Design review of the part built by this model. Coordinates are the model's own, in mm. Face numbers are marked on the shaded views. A direction names the side the tool comes from. Coordinates: 2 decimals unless noted, no trailing zeros. Order: outer loops, then holes, each group sorted by start corner. A loop starts at its lowest first (then second) coordinate and runs counter-clockwise, first axis right, second up. Notation, with made-up numbers: (30, 37.25) -> (88, 37.25) arc R32 ccw to (88, 66.25) -> close; hole circle Ø6 at (1.25, 28). An arc over 180 degrees is marked (long way). Write item = value, one per line.
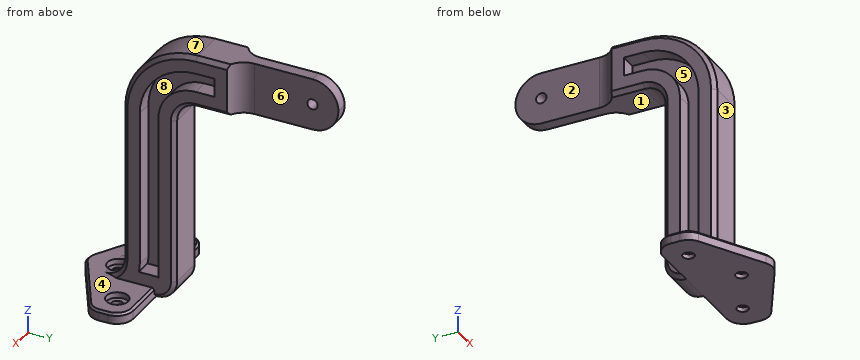
```python
from build123d import *

# Parameters (mm, degrees)
BOSS_EXTRUDE1_DEPTH             = 5
FILLET1_R                       = 8
CBORE_FOR_M5_SBHCS1_D           = 5.5
CBORE_FOR_M5_SBHCS1_DEPTH       = 10
CBORE_FOR_M5_SBHCS1_CBORE_D     = 10.5
CBORE_FOR_M5_SBHCS1_CBORE_DEPTH = 2.75
CBORE_FOR_M5_SBHCS1_TIP         = 1.652366702
SKETCH7_W                       = 20
SKETCH7_H                       = 100
BOSS_EXTRUDE2_DEPTH             = 120
SKETCH8_W                       = 190
SKETCH8_H                       = 150
CUT_EXTRUDE1_DEPTH              = 72
FILLET2_R                       = 12.5
SKETCH9_W                       = 14.25
SKETCH9_H                       = 100
CUT_EXTRUDE2_DEPTH              = 72
SKETCH10_R                      = 2.5
CUT_EXTRUDE3_DEPTH              = 72
FILLET3_R                       = 10
FILLET4_R                       = 10
FILLET5_R                       = 35
FILLET6_R                       = 10
SKETCH12_W                      = 20
SKETCH12_H                      = 10
BOSS_EXTRUDE3_DEPTH             = 5
FILLET7_R                       = 10
CHAMFER1_SIZE                   = 2
CHAMFER2_SIZE                   = 1
CUT_EXTRUDE4_DEPTH              = 8


# Some blends are built 0.0001 mm under size
with BuildPart() as part:
    # Sketch2 → Boss-Extrude1 (new body)
    with BuildSketch(Plane.XY):
        Polygon((-37.5, 28.000635095), (0, 6.35), (37.5, 28.000635095), (37.5, 45), (-37.5, 45), align=None)
    extrude(amount=BOSS_EXTRUDE1_DEPTH)

    # Fillet1
    fillet1_edges = [part.edges().sort_by_distance(p)[0] for p in [
        (37.5, 28.000635095, 2.5),
        (0, 6.35, 2.5),
        (-37.5, 28.000635095, 2.5),
        (-37.5, 45, 2.5),
        (37.5, 45, 2.5),
    ]]
    fillet(fillet1_edges, radius=FILLET1_R)

    # CBORE for M5 SBHCS1
    with Locations(Plane.XY.offset(5)):
        with Locations((-25, 35), (0, 22.5), (25, 35)):
            CounterBoreHole(CBORE_FOR_M5_SBHCS1_D / 2, CBORE_FOR_M5_SBHCS1_CBORE_D / 2, CBORE_FOR_M5_SBHCS1_CBORE_DEPTH, depth=CBORE_FOR_M5_SBHCS1_DEPTH)
            with Locations((0, 0, -(CBORE_FOR_M5_SBHCS1_DEPTH + CBORE_FOR_M5_SBHCS1_TIP / 2))):  # 118° drill point
                Cone(0, CBORE_FOR_M5_SBHCS1_D / 2, CBORE_FOR_M5_SBHCS1_TIP, mode=Mode.SUBTRACT)

    # Sketch7 → Boss-Extrude2 (add)
    with BuildSketch(Plane.XY.offset(5)):
        with Locations((0, 80)):
            Rectangle(SKETCH7_W, SKETCH7_H)
    extrude(amount=BOSS_EXTRUDE2_DEPTH)

    # Sketch8 → Cut-Extrude1 (cut)
    with BuildSketch(Plane(origin=(10, 0, 0), x_dir=(0, 0, -1), z_dir=(1, 0, 0))):
        with Locations((-5, 130)):
            Rectangle(SKETCH8_W, SKETCH8_H)
    extrude(amount=-CUT_EXTRUDE1_DEPTH, mode=Mode.SUBTRACT)

    # Fillet2
    fillet2_edges = [part.edges().sort_by_distance(p)[0] for p in [
        (0, 130, 100),
        (0, 130, 125),
    ]]
    fillet(fillet2_edges, radius=FILLET2_R - 0.0001)  # a hair under: the kernel refuses the full size

    # Sketch9 → Cut-Extrude2 (cut)
    with BuildSketch(Plane.XY.offset(125)):
        with Locations((10, 130)):
            Rectangle(SKETCH9_W, SKETCH9_H)
        with Locations((-10, 130)):
            Rectangle(SKETCH9_W, SKETCH9_H)
    extrude(amount=-CUT_EXTRUDE2_DEPTH, mode=Mode.SUBTRACT)

    # Sketch10 → Cut-Extrude3 (cut)
    with BuildSketch(Plane(origin=(2.875, 0, 0), x_dir=(0, 0, -1), z_dir=(1, 0, 0))):
        with Locations((-112.5, 117.5)):
            Circle(SKETCH10_R)
    extrude(amount=-CUT_EXTRUDE3_DEPTH, mode=Mode.SUBTRACT)

    # Fillet3
    # the kernel refuses this fillet: 10 mm, written as the material it adds along each edge
    with BuildSketch(Plane(origin=(-2.875, 80, 125), x_dir=(-1, 0, 0), z_dir=(0, 0, -1))) as fillet3_piece_1:
        with BuildLine():
            CenterArc((10, 9.577806377), FILLET3_R, 180, 73.291656284)
            Line((0, 9.577806377), (-0.2, 9.577806377))
            Line((-0.2, 9.577806377), (-0.2, 0))
            Line((-0.2, 0), (0, -0.2))
            ThreePointArc((0, -0.2), (3.5625, -0.2), (7.0675, -0.191556128))
            Line((7.0675, -0.191556128), (7.125, 0))
        make_face()
    extrude(amount=25)
    with BuildSketch(Plane(origin=(2.875, 80, 125), x_dir=(0, 1, 0), z_dir=(0, 0, -1))) as fillet3_piece_2:
        with BuildLine():
            CenterArc((9.577806377, 10), FILLET3_R, 196.708343716, 73.291656284)
            Line((0, 7.125), (-0.191556128, 7.0675))
            ThreePointArc((-0.191556128, 7.0675), (-0.2, 3.5625), (-0.2, 0))
            Line((-0.2, 0), (0, -0.2))
            Line((0, -0.2), (9.577806377, -0.2))
            Line((9.577806377, -0.2), (9.577806377, 0))
        make_face()
    extrude(amount=25)

    # Fillet4
    fillet4_edges = [part.edges().sort_by_distance(p)[0] for p in [
        (0, 55, 100),
    ]]
    fillet(fillet4_edges, radius=FILLET4_R)

    # Fillet5
    fillet5_edges = [part.edges().sort_by_distance(p)[0] for p in [
        (0, 30, 125),
    ]]
    fillet(fillet5_edges, radius=FILLET5_R)

    # Fillet6
    # the kernel refuses this fillet: 10 mm, written as the material it adds along each edge
    with BuildSketch(Plane(origin=(10, 30, 5), x_dir=(0, 0, 1), z_dir=(-1, 0, 0))) as fillet6_piece_1_section:
        with BuildLine():
            CenterArc((FILLET6_R, -FILLET6_R), FILLET6_R, 90, 90)
            Line((0, -FILLET6_R), (0, 0))
            Line((0, 0), (FILLET6_R, 0))
        make_face()
    fillet6_piece_1 = extrude(amount=20, mode=Mode.PRIVATE)
    fillet6_piece_1 = fillet6_piece_1 - Plane(origin=(0, 22.5, 7.53044348), x_dir=(1, 0, 0), z_dir=(0, 0, 1)) * Cylinder(5.25, 80, mode=Mode.PRIVATE)
    add(fillet6_piece_1)

    # Sketch12 → Boss-Extrude3 (add)
    with BuildSketch(Plane(origin=(0, 0, 5), x_dir=(-1, 0, 0), z_dir=(0, 0, -1))):
        with Locations((0, 50)):
            Rectangle(SKETCH12_W, SKETCH12_H)
    extrude(amount=BOSS_EXTRUDE3_DEPTH)

    # Fillet7
    # the kernel refuses this fillet: 10 mm, written as the material it takes off along each edge
    with BuildSketch(Plane(origin=(-35, 55, 0), x_dir=(0, 0, 1), z_dir=(1, 0, 0))) as fillet7_piece_1:
        with BuildLine():
            CenterArc((FILLET7_R, FILLET7_R), FILLET7_R, 180, 90)
            Line((0, FILLET7_R), (0, 0))
            Line((0, 0), (FILLET7_R, 0))
        make_face()
    extrude(amount=70, mode=Mode.SUBTRACT)

    # Chamfer1
    # the kernel refuses this chamfer: 2 mm, written as the material it takes off along each edge
    with BuildSketch(Plane(origin=(-10, 65, 100), x_dir=(-0.02749587661058987, 0, 0.9996219169112968), z_dir=(0, 1, 0)), Plane(origin=(10, 85.143365976, 100), x_dir=(0.027495876610586414, 0, 0.9996219169112968), z_dir=(0, -1, 0))) as chamfer1_piece_1:
        Polygon((CHAMFER1_SIZE * 0.999621916911, CHAMFER1_SIZE * 0.0274958766106), (-CHAMFER1_SIZE * 0.0274958766106, CHAMFER1_SIZE * 0.999621916911), (0, 0), align=None)
    extrude(amount=20.143365976, mode=Mode.SUBTRACT)
    with BuildSketch(Plane(origin=(-10, 65, 125), x_dir=(-0.02749587661058987, 0, -0.9996219169112968), z_dir=(0, 1, 0)), Plane(origin=(10, 85.143365976, 125), x_dir=(0.027495876610586414, 0, -0.9996219169112968), z_dir=(0, -1, 0))) as chamfer1_piece_2:
        Polygon((CHAMFER1_SIZE * 0.999621916911, -CHAMFER1_SIZE * 0.0274958766106), (-CHAMFER1_SIZE * 0.0274958766106, -CHAMFER1_SIZE * 0.999621916911), (0, 0), align=None)
    extrude(amount=20.143365976, mode=Mode.SUBTRACT)
    with BuildSketch(Plane(origin=(-10, 55, 10), x_dir=(-0.027495876610589956, -0.9996219169112965, 0), z_dir=(0, 0, 1)), Plane(origin=(10, 55, 90), x_dir=(0.0274958766105822, -0.999621916911297, 0), z_dir=(0, 0, -1))) as chamfer1_piece_3:
        Polygon((CHAMFER1_SIZE * 0.999621916911, CHAMFER1_SIZE * 0.0274958766106), (-CHAMFER1_SIZE * 0.0274958766106, CHAMFER1_SIZE * 0.999621916911), (0, 0), align=None)
    extrude(amount=80, mode=Mode.SUBTRACT)
    with BuildSketch(Plane(origin=(10, 65, 90), x_dir=(0, 0, 1), z_dir=(0, 1, 0))) as chamfer1_piece_4:
        Polygon((10 + CHAMFER1_SIZE, 0), (10, -CHAMFER1_SIZE), (10, 0), align=None)
    revolve(axis=Axis((10, 65, 90), (1, 0, 0)), revolution_arc=90, mode=Mode.SUBTRACT)
    with BuildSketch(Plane(origin=(-10, 65, 90), x_dir=(0, 0, 1), z_dir=(0, 1, 0))) as chamfer1_piece_5:
        Polygon((10 + CHAMFER1_SIZE, 0), (10, CHAMFER1_SIZE), (10, 0), align=None)
    revolve(axis=Axis((-10, 65, 90), (1, 0, 0)), revolution_arc=90, mode=Mode.SUBTRACT)
    with BuildSketch(Plane(origin=(10, 30, 15), x_dir=(0.027495876610581334, 0.999621916911297, 0), z_dir=(0, 0, 1)), Plane(origin=(-10, 30, 15), x_dir=(0.9996219169112968, -0.027495876610585623, 0), z_dir=(0, 0, 1))) as chamfer1_piece_6:
        Polygon((CHAMFER1_SIZE * 0.999621916911, CHAMFER1_SIZE * 0.0274958766106), (-CHAMFER1_SIZE * 0.0274958766106, CHAMFER1_SIZE * 0.999621916911), (0, 0), align=None)
    extrude(amount=75, mode=Mode.SUBTRACT)
    with BuildSketch(Plane(origin=(10, 65, 90), x_dir=(0, 0, 1), z_dir=(0, 1, 0))) as chamfer1_piece_7:
        Polygon((35 - CHAMFER1_SIZE, 0), (35, -CHAMFER1_SIZE), (35, 0), align=None)
    revolve(axis=Axis((10, 65, 90), (1, 0, 0)), revolution_arc=90, mode=Mode.SUBTRACT)
    with BuildSketch(Plane(origin=(-10, 65, 90), x_dir=(0, 0, 1), z_dir=(0, 1, 0))) as chamfer1_piece_8:
        Polygon((35 - CHAMFER1_SIZE, 0), (35, CHAMFER1_SIZE), (35, 0), align=None)
    revolve(axis=Axis((-10, 65, 90), (1, 0, 0)), revolution_arc=90, mode=Mode.SUBTRACT)
    with BuildSketch(Plane(origin=(10, 20, 15), x_dir=(0, 1, 0), z_dir=(0, 0, 1))) as chamfer1_piece_9_section:
        Polygon((10, CHAMFER1_SIZE), (10 + CHAMFER1_SIZE, 0), (10, 0), align=None)
    chamfer1_piece_9 = revolve(axis=Axis((10, 20, 15), (-1, 0, 0)), revolution_arc=119.481154356, mode=Mode.PRIVATE)
    chamfer1_piece_9 = split(chamfer1_piece_9, bisect_by=Plane(origin=(9.27752792, 27.153705444, 5), z_dir=(0, 0, 1)), keep=Keep.TOP, mode=Mode.PRIVATE)
    add(chamfer1_piece_9, mode=Mode.SUBTRACT)
    with BuildSketch(Plane(origin=(-10, 20, 15), x_dir=(0, 1, 0), z_dir=(0, 0, 1))) as chamfer1_piece_10_section:
        Polygon((10, -CHAMFER1_SIZE), (10 + CHAMFER1_SIZE, 0), (10, 0), align=None)
    chamfer1_piece_10 = revolve(axis=Axis((-10, 20, 15), (-1, 0, 0)), revolution_arc=119.481154356, mode=Mode.PRIVATE)
    chamfer1_piece_10 = split(chamfer1_piece_10, bisect_by=Plane(origin=(-9.27752792, 27.153705444, 5), z_dir=(0, 0, 1)), keep=Keep.TOP, mode=Mode.PRIVATE)
    add(chamfer1_piece_10, mode=Mode.SUBTRACT)
    with BuildSketch(Plane(origin=(10, 45, 10), x_dir=(0, 1, 0), z_dir=(0, 0, 1))) as chamfer1_piece_11:
        Polygon((10 - CHAMFER1_SIZE, 0), (10, CHAMFER1_SIZE), (10, 0), align=None)
    revolve(axis=Axis((10, 45, 10), (-1, 0, 0)), revolution_arc=90, mode=Mode.SUBTRACT)
    with BuildSketch(Plane(origin=(-10, 45, 10), x_dir=(0, 1, 0), z_dir=(0, 0, 1))) as chamfer1_piece_12:
        Polygon((10 - CHAMFER1_SIZE, 0), (10, -CHAMFER1_SIZE), (10, 0), align=None)
    revolve(axis=Axis((-10, 45, 10), (-1, 0, 0)), revolution_arc=90, mode=Mode.SUBTRACT)

    # Chamfer2
    chamfer2_edges = [part.edges().sort_by_distance(p)[0] for p in [
        (-37.5, 34.809718624, 5),
        (19.75, 45, 5),
        (37.5, 34.809718624, 5),
        (-18.75, 17.175317547, 5),
        (18.75, 17.175317547, 5),
        (35.156854249, 42.656854249, 5),
        (36.42820323, 28.619437248, 5),
        (0, 7.587604307, 5),
        (-36.42820323, 28.619437248, 5),
        (-35.156854249, 42.656854249, 5),
        (-19.75, 45, 5),
    ]]
    chamfer(chamfer2_edges, length=CHAMFER2_SIZE)

    # Sketch13 → Cut-Extrude4 (cut)
    with BuildSketch(Plane(origin=(10, 0, 0), x_dir=(0, 0, -1), z_dir=(1, 0, 0))):
        with BuildLine():
            Line((-11, 37.549928775), (-11, 46.485281374))
            Line((-11, 46.485281374), (-10.485281374, 47))
            Line((-10.485281374, 47), (-90, 47))
            ThreePointArc((-90, 47), (-102.727922061, 52.272077939), (-108, 65))
            Line((-108, 65), (-108, 74))
            Line((-108, 74), (-117, 74))
            Line((-117, 74), (-117, 65))
            ThreePointArc((-117, 65), (-109.091883092, 45.908116908), (-90, 38))
            Line((-90, 38), (-15, 38))
            ThreePointArc((-15, 38), (-12.987379562, 37.887128304), (-11, 37.549928775))
        make_face()
    cut_extrude4 = extrude(amount=-CUT_EXTRUDE4_DEPTH, mode=Mode.SUBTRACT)

    # Mirror1: Cut-Extrude4 across plane
    add(cut_extrude4.mirror(Plane(origin=(0, 0, 0), x_dir=(0, 0, 1), z_dir=(1, 0, 0))), mode=Mode.SUBTRACT)


solid = part.part
```
(1) For the marked faces 1, 2, 3, 4 and 5, list the 3-axis set-ups (+Z, -Z, +X, -X, +Y, -Y) from which the entire face can be reached by the end or side of a thin tool; tool diameter is ignored.
Report:
face_1 = -Z, +X, -X, +Y
face_2 = +Z, -Z, -X, +Y
face_3 = +Z, +X, -X, -Y
face_4 = +Z, -Y
face_5 = -X
(2) The part is to be moulded in two halves that separate along Y. For the marked faces 6, 7 and 8, say which applies: released by +Y, released by -Y, zero draft, split by the parting line, or undercut.
Report:
face_6 = zero draft
face_7 = released by -Y
face_8 = undercut
(3) We need section A-A (x = 0). Give the number of separate pieces and of enclosed holes in the cut face, and give its area (3 significant figures).
Report:
separate_pieces = 2
enclosed_holes = 1
area = 4,730 mm²
(4) We need section C-C (x = 25). Write out the cut boundary in (y, z), and give its area (3 significant figures).
Report:
outline = (20.78, 0) -> (32.25, 0) -> (32.25, 2.25) -> (29.75, 2.25) -> (29.75, 5) -> (21.94, 5) -> (20.78, 4) -> close; (37.75, 0) -> (45, 0) -> (45, 4) -> (44, 5) -> (40.25, 5) -> (40.25, 2.25) -> (37.75, 2.25) -> close
area = 78.8 mm²
(5) We need section D-D (y = 94). Write out the cut boundary in (x, z) (3 decimals), and give its area (3 significant figures).
Report:
outline = (-2.875, 100) -> (2.875, 100) -> (2.875, 125) -> (-2.875, 125) -> close
area = 144 mm²
(6) Insertion check: pin 1 (8.5 mm diameter, centred on x = 25, y = 35, fed in from +Z); pin 2 (1 mm diameter, centred on x = -2, y = 70.5, fed in from -Z); pin 3 (8 mm diameter, centred on x = -3.5, z = 61.5, fed in from +Y). Each pin has a flat end and moves straight along its axis. Give the tip position at first contact, or say it passes through.
Report:
pin_1 = 2.25
pin_2 = 100
pin_3 = 55
(7) We need section B-B (z = 67). Write out the cut boundary in (x, y).
Report:
outline = (-10, 32) -> (-8, 30) -> (8, 30) -> (10, 32) -> (10, 38) -> (2, 38) -> (2, 47) -> (10, 47) -> (10, 53) -> (8, 55) -> (-8, 55) -> (-10, 53) -> (-10, 47) -> (-2, 47) -> (-2, 38) -> (-10, 38) -> close
(8) For L1, parallel to Y at x = 2.5, z = 75.5; L2, parallel to X at y = 74, z = 107.5; L3, parallel to Z at x = -25, y = 28, list the stretches that pass through material, from the lowest coordinate up.
Report:
L1 = 30 to 38, 47 to 55
L2 = -10 to 10
L3 = 0 to 5
